```python
from build123d import *

# Parameters (mm, degrees)
SKETCH1_R           = 0.5
SKETCH1_R_2         = 2
SKETCH1_R_3         = 1
SKETCH1_R_4         = 1.5
BOSS_EXTRUDE1_DEPTH = 1
SKETCH1_4_R         = 2
BOSS_EXTRUDE2_DEPTH = 3


with BuildPart() as part:
    # Sketch1 → Boss-Extrude1 (new body)
    # profile 1 of 6: a face of its own
    with BuildSketch(Plane(origin=(0, 0, 0), x_dir=(1, 0, 0), z_dir=(0, 1, 0))):
        with BuildLine():
            ThreePointArc((-0.4315197, -2.462476548), (-2.5, 0), (-0.4315197, 2.462476548))
            Line((-0.4315197, 2.462476548), (-11.5, 1.5))
            ThreePointArc((-11.5, 1.5), (-10.439339828, 1.060660172), (-10, 0))
            ThreePointArc((-10, 0), (-10.439339828, -1.060660172), (-11.5, -1.5))
            Line((-11.5, -1.5), (-0.4315197, -2.462476548))
        make_face()
        with Locations(Location((-9, 0, 0), (0, 0, 270))):
            Circle(SKETCH1_R, mode=Mode.SUBTRACT)
        with Locations(Location((-6.5, 0, 0), (0, 0, 270))):
            Circle(SKETCH1_R, mode=Mode.SUBTRACT)
    # profile 2 of 6: a face of its own
    with BuildSketch(Plane(origin=(0, 0, 0), x_dir=(1, 0, 0), z_dir=(0, 1, 0))):
        with BuildLine():
            ThreePointArc((2.5, 0), (1.914262162, 1.607980216), (0.4315197, 2.462476548))
            Line((0.4315197, 2.462476548), (0, 2.5))
            Line((0, 2.5), (-0.4315197, 2.462476548))
            ThreePointArc((-0.4315197, 2.462476548), (-2.5, 0), (-0.4315197, -2.462476548))
            Line((-0.4315197, -2.462476548), (0, -2.5))
            Line((0, -2.5), (0.4315197, -2.462476548))
            ThreePointArc((0.4315197, -2.462476548), (1.914262162, -1.607980216), (2.5, 0))
        make_face()
        Circle(SKETCH1_R_2, mode=Mode.SUBTRACT)
    # profile 3 of 6: a face of its own
    with BuildSketch(Plane(origin=(0, 0, 0), x_dir=(1, 0, 0), z_dir=(0, 1, 0))):
        Circle(SKETCH1_R_2)
        with Locations(Location((0, 0, 0), (0, 0, 270))):
            Circle(SKETCH1_R_3, mode=Mode.SUBTRACT)
    # profile 4 of 6: a face of its own
    with BuildSketch(Plane(origin=(0, 0, 0), x_dir=(1, 0, 0), z_dir=(0, 1, 0))):
        with BuildLine():
            ThreePointArc((11.5, -1.5), (10, 0), (11.5, 1.5))
            Line((11.5, 1.5), (0.4315197, 2.462476548))
            ThreePointArc((0.4315197, 2.462476548), (1.914262162, 1.607980216), (2.5, 0))
            ThreePointArc((2.5, 0), (1.914262162, -1.607980216), (0.4315197, -2.462476548))
            Line((0.4315197, -2.462476548), (11.5, -1.5))
        make_face()
        with Locations(Location((6.5, 0, 0), (0, 0, 270))):
            Circle(SKETCH1_R, mode=Mode.SUBTRACT)
        with Locations(Location((9, 0, 0), (0, 0, 270))):
            Circle(SKETCH1_R, mode=Mode.SUBTRACT)
    # profile 5 of 6: a face of its own
    with BuildSketch(Plane(origin=(0, 0, 0), x_dir=(1, 0, 0), z_dir=(0, 1, 0))):
        with Locations((11.5, 0)):
            Circle(SKETCH1_R_4)
        with Locations(Location((11.5, 0, 0), (0, 0, 270))):
            Circle(SKETCH1_R, mode=Mode.SUBTRACT)
    # profile 6 of 6: a face of its own
    with BuildSketch(Plane(origin=(0, 0, 0), x_dir=(1, 0, 0), z_dir=(0, 1, 0))):
        with Locations((-11.5, 0)):
            Circle(SKETCH1_R_4)
        with Locations(Location((-11.5, 0, 0), (0, 0, 270))):
            Circle(SKETCH1_R, mode=Mode.SUBTRACT)
    extrude(amount=BOSS_EXTRUDE1_DEPTH)

    # Sketch1_4 → Boss-Extrude2 (add)
    with BuildSketch(Plane(origin=(0, 0, 0), x_dir=(1, 0, 0), z_dir=(0, 1, 0))):
        with BuildLine():
            ThreePointArc((2.5, 0), (1.914262162, 1.607980216), (0.4315197, 2.462476548))
            Line((0.4315197, 2.462476548), (0, 2.5))
            Line((0, 2.5), (-0.4315197, 2.462476548))
            ThreePointArc((-0.4315197, 2.462476548), (-2.5, 0), (-0.4315197, -2.462476548))
            Line((-0.4315197, -2.462476548), (0, -2.5))
            Line((0, -2.5), (0.4315197, -2.462476548))
            ThreePointArc((0.4315197, -2.462476548), (1.914262162, -1.607980216), (2.5, 0))
        make_face()
        with Locations(Location((0, 0, 0), (0, 0, 270))):
            Circle(SKETCH1_4_R, mode=Mode.SUBTRACT)
    extrude(amount=BOSS_EXTRUDE2_DEPTH)


solid = part.part
```
Could you check a few things on this model? Use its own coordinates, in mm. A direction names the side the tool comes from. Round coordinates to 2 decimals unless told otherwise and drop trailing zeros. Order: outer loops, then holes, each group sorted by start corner. A loop starts at its lowest first (then second) coordinate and runs counter-clockwise, first axis right, second up. Notation, with made-up numbers: M 73.25,31.25 L 106.25,31.25 A36 ccw 106.25,70.25 Z; hole C -3,26 d10. An arc over 180 degrees is marked long. One line per question, with ' | ' between items. Start each with the question number.
(1) Suppose I cut it at C-C on y = 0.45. List the corners of the cut face in (x, z) for me, then the cut area to 3 significant figures.
(2) For faces 4 (the face through (-0.976, 0.493, -0.217)), 5 (the face through (-2.5, 2, 0)), 6 (the face through (-2, 2, 0)), which set-ups out of +Z, -Z, +X, -X, +Y, -Y let a thin tool reach every point of the face, with its end or its side?
(3) Please list where these lines run through material, in increasing order: line 1 along Z through (x, y) = (0.5, 1.9); line 2 along X through (y, z) = (2.15, 1.5).
(4) Suppose I cut it at B-B on z = 0.75. List the corners of the cut face in (x, y) for me.
(5) Suppose I cut it at A-A on y = 2.6. List the corners of the cut face in (x, z) for me.
(6) Suppose I cut it at D-D on x = -6.5. List the corners of the cut face in (y, z) for me.
(7) Thinking about a two-plate mould opening in Z: for faces 1 (the face through (-7, 1, -1)), 2 (the face through (8.512, 0.493, -0.108)), 3 (the face through (-13, 0.5, 0)), which applies, +Z half, -Z half, draft (parallel to the pull), parting line (faces both ways), or undercut?
(8) For P1, Ø2.5, axis at x = 8.5, z = -1, coming from the +Y side; P2, Ø1, axis at x = 10.5, y = 0.5, coming from the +Z side, each with a flat end and sliding along its axis, tell me the tip position at first contact or that it passes through.
Geometry results:
1) outline: M -11.5,-1.5 L 0,-2.5 L 11.5,-1.5 A1.5 ccw 11.5,1.5 L 0,2.5 L -11.5,1.5 A1.5 ccw Z; hole C -11.5,0 d1; hole C -9,0 d1; hole C -6.5,0 d1; hole C 0,0 d2; hole C 6.5,0 d1; hole C 9,0 d1; hole C 11.5,0 d1 | area: 91.2 mm²
2) face 4: +Y, -Y | face 5: -X, +Y | face 6: +Y
3) line 1: -2.45 to -1.94, 1.94 to 2.45 | line 2: -2 to -1.32, 1.32 to 2
4) outline: M -12.8,0 L -0.66,0 L -0.66,1 L -1.85,1 L -1.85,3 L -2.38,3 L -2.38,1 L -12.8,1 Z; M 0.66,0 L 12.8,0 L 12.8,1 L 2.38,1 L 2.38,3 L 1.85,3 L 1.85,1 L 0.66,1 Z
5) outline: M -0.43,-2.46 L 0,-2.5 L 0.43,-2.46 A2.5 ccw 0.43,2.46 L 0,2.5 L -0.43,2.46 A2.5 ccw Z; hole C 0,0 d4
6) outline: M 0,-1.93 L 1,-1.93 L 1,-0.5 L 0,-0.5 Z; M 0,0.5 L 1,0.5 L 1,1.93 L 0,1.93 Z
7) face 1: draft | face 2: undercut | face 3: parting line
8) P1: y = 1 | P2: z = 1.63
